Source: CAD feature listing. Evaluate the final solid. Frame: model axes, mm. Face numbers are marked on the shaded views. A direction names the side the tool comes from. Give positions to 0.01 mm unless a question says otherwise; leave off trailing zeros. Loops run counter-clockwise (first coordinate to the right, second up) from the corner with the lowest first, then second, coordinate; pieces in that order, holes last. Notation, with made-up numbers: M -29,-15.5 L -19,-15.5 A14 cw -19,8.5 Z; hole C 36,-7 d5. An arc over 180 degrees is marked long. Put each result on its own line as item: value.
from build123d import *

# Parameters (mm, degrees)
SKETCH2_W           = 17
SKETCH2_H           = 3.5
SKETCH2_H_2         = 6.75
BOSS_EXTRUDE1_DEPTH = 4
SKETCH3_R           = 7.15
BOSS_EXTRUDE2_DEPTH = 5.3
SKETCH4_R           = 9
BOSS_EXTRUDE3_DEPTH = 12.3
SKETCH5_R           = 8.3
BOSS_EXTRUDE4_DEPTH = 5.3


with BuildPart() as part:
    # Sketch2 → Boss-Extrude1 (new body)
    with BuildSketch(Plane.XY):
        Rectangle(SKETCH2_W, SKETCH2_H)
        with BuildLine():
            Line((-9, -1.75), (-8.5, -1.75))
            Line((-8.5, -1.75), (-8.5, 1.75))
            Line((-8.5, 1.75), (-9, 1.75))
            ThreePointArc((-9, 1.75), (-10.75, 0), (-9, -1.75))
        make_face()
        with Locations((0, 5.125)):
            Rectangle(SKETCH2_W, SKETCH2_H_2)
        with Locations((0, -5.125)):
            Rectangle(SKETCH2_W, SKETCH2_H_2)
        with BuildLine():
            Line((8.5, 1.75), (8.5, -1.75))
            Line((8.5, -1.75), (9, -1.75))
            ThreePointArc((9, -1.75), (10.75, 0), (9, 1.75))
            Line((9, 1.75), (8.5, 1.75))
        make_face()
    extrude(amount=BOSS_EXTRUDE1_DEPTH)

    # Sketch3 → Boss-Extrude2 (add)
    with BuildSketch(Plane.XY.offset(4)):
        Circle(SKETCH3_R)
    extrude(amount=BOSS_EXTRUDE2_DEPTH)

    # Sketch4 → Boss-Extrude3 (add)
    with BuildSketch(Plane.XY.offset(9.3)):
        Circle(SKETCH4_R)
    extrude(amount=BOSS_EXTRUDE3_DEPTH)

    # Sketch5 → Boss-Extrude4 (add)
    with BuildSketch(Plane.XY.offset(21.6)):
        Circle(SKETCH5_R)
    extrude(amount=BOSS_EXTRUDE4_DEPTH)


solid = part.part
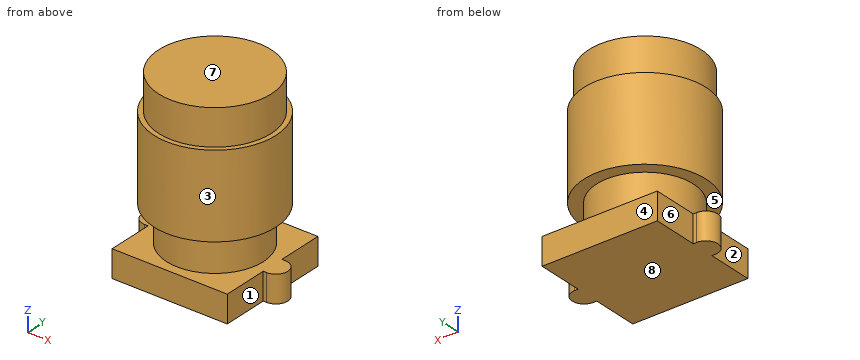
1. Material intervals for line 1 (Z direction, x = -8.75, y = -1.5); line 2 (Z direction, x = -7, y = -4); line 3 (Z direction, x = 7.5, y = 5.25), sorted ascending. Write a range as from..to.
Found:
line 1: 0..4, 9.3..21.6
line 2: 0..4, 9.3..26.9
line 3: 0..4
2. Contact query for flat-ended pins moving along their axis: P1, Ø3, axis at y = -4.5, z = 2, coming from the +X side; P2, Ø4, axis at y = 3, z = 22.5, coming from the -X side; P3, Ø4.5, axis at y = -6.5, z = 2, coming from the -X side. Output: stop coordinate, or through.
Found:
P1: x = 8.5
P2: x = -8.92
P3: x = -8.5
3. Section query A-A (x = 0). Output: boundary loops of the cut face in (y, z), plus the area to 3 significant figures.
Found:
outline: M -9,9.3 L -7.15,9.3 L -7.15,4 L -8.5,4 L -8.5,0 L 8.5,0 L 8.5,4 L 7.15,4 L 7.15,9.3 L 9,9.3 L 9,21.6 L 8.3,21.6 L 8.3,26.9 L -8.3,26.9 L -8.3,21.6 L -9,21.6 Z
area: 453 mm^2
4. Section query B-B (z = 2). Output: boundary loops of the cut face in (x, y).
Found:
outline: M -9,-1.75 L -8.5,-1.75 L -8.5,-8.5 L 8.5,-8.5 L 8.5,-1.75 L 9,-1.75 A1.75 ccw 9,1.75 L 8.5,1.75 L 8.5,8.5 L -8.5,8.5 L -8.5,1.75 L -9,1.75 A1.75 ccw Z
5. Draft query along Z for the marked faces 5, 6, 7 and 8. Return one class per face: pulls with the +Z half, pulls with the -Z half, needs draft (parallel to the pull), parting line crosses it, or undercut.
Found:
face 5: undercut
face 6: needs draft
face 7: pulls with the +Z half
face 8: pulls with the -Z half
6. Section query D-D (y = 5.5). Output: boundary loops of the cut face in (x, z).
Found:
outline: M -8.5,0 L 8.5,0 L 8.5,4 L 4.57,4 L 4.57,9.3 L 7.12,9.3 L 7.12,21.6 L 6.22,21.6 L 6.22,26.9 L -6.22,26.9 L -6.22,21.6 L -7.12,21.6 L -7.12,9.3 L -4.57,9.3 L -4.57,4 L -8.5,4 Z
7. Section query C-C (y = -7.5). Output: boundary loops of the cut face in (x, z).
Found:
outline: M -8.5,0 L 8.5,0 L 8.5,4 L -8.5,4 Z; M -4.97,9.3 L 4.97,9.3 L 4.97,21.6 L 3.56,21.6 L 3.56,26.9 L -3.56,26.9 L -3.56,21.6 L -4.97,21.6 Z
8. Access query for the marked faces 1, 2, 3 and 4. Directions: +Z, -Z, +X, -X, +Y, -Y. A direction counts if a zero-diameter tool reaches every point of the face in a straight line with its end or side. Return the directions, or none.
Found:
face 1: -Z, +X, -Y
face 2: -Z, -X, -Y
face 3: +Z
face 4: -Z, +X, -X, +Y
